```python
from build123d import *

# Parameters (mm, degrees)
F0_W     = 117
F0_H     = 15
F0_R     = 0.5
F1_DEPTH = 20
F2_W     = 10
F2_H     = 10
F3_DEPTH = 37


with BuildPart() as f1:
    # F0 (on Front) → F1 (new body)
    with BuildSketch(Plane.XZ):
        with Locations((67, 12)):
            Rectangle(F0_W, F0_H)
        with Locations((16, 12)):
            Circle(F0_R, mode=Mode.SUBTRACT)
        with Locations((40, 12)):
            Circle(F0_R, mode=Mode.SUBTRACT)
        with Locations((76, 12)):
            Circle(F0_R, mode=Mode.SUBTRACT)
        with Locations((106, 12)):
            Circle(F0_R, mode=Mode.SUBTRACT)
        with Locations((118, 12)):
            Circle(F0_R, mode=Mode.SUBTRACT)
    extrude(amount=F1_DEPTH)

    # F2 (on face) → F3 (cut)
    with BuildSketch(Plane.XY.offset(19.5)):
        with Locations((40, -10)):
            Rectangle(F2_W, F2_H)
        with Locations((106, -10)):
            Rectangle(F2_W, F2_H)
    extrude(amount=-F3_DEPTH, mode=Mode.SUBTRACT)


solid = f1.part
```
Here's how the part is built. I have some questions about the finished solid (model axes, mm). A direction names the side the tool comes from. Coordinates: 2 decimals unless noted, no trailing zeros. Order: outer loops, then holes, each group sorted by start corner. A loop starts at its lowest first (then second) coordinate and runs counter-clockwise, first axis right, second up.
1) Imagine slicing it at A-A on y = -9.25. List the corners of the cut face in (x, z) for me.
2) We'd pull the mould along Y, two halves only. Please class faces 1 (the face through (8.5, -10, 12)), 2 (the face through (41, -15, 12)), 3 (the face through (41, -5, 12)), 4 (the face through (66, 0, 12)): +Y half, -Y half, draft (parallel to the pull), parting line (faces both ways), or undercut.
3) Will this pin go through, and if not, where does the flat tip stop? pin 1 (8 mm diameter, centred on x = 41.5, z = 11.5, fed in from +Y).
4) I need wall thicknesses on line 1 (Z direction, x = 40, y = -4); line 2 (X direction, y = -5.25, z = 15); line 3 (Y direction, x = 109.5, z = 10.5). Which ranges of each line are inside material? Lowest first, please.
5) Which directions (+Z, -Z, +X, -X, +Y, -Y) give clear straight access to the entire face, cutting with the end or side of a thin tool? Please do faces 5 (the face through (66, -20, 12)), 6 (the face through (35, -10, 12)).
6) Imagine slicing it at B-B on z = 6.5. List the corners of the cut face in (x, y) for me, and give its area (3 significant figures).
Response values:
1. outline: (8.5, 4.5) - (35, 4.5) - (35, 19.5) - (8.5, 19.5) - close; (45, 4.5) - (101, 4.5) - (101, 19.5) - (45, 19.5) - close; (111, 4.5) - (125.5, 4.5) - (125.5, 19.5) - (111, 19.5) - close; hole circle Ø1 at (16, 12); hole circle Ø1 at (76, 12); hole circle Ø1 at (118, 12)
2. face 1: draft
2. face 2: undercut
2. face 3: undercut
2. face 4: +Y half
3. pin 1: stops at y = 0
4. line 1: z = 4.5 to 11.5, 12.5 to 19.5
4. line 2: x = 8.5 to 35, 45 to 101, 111 to 125.5
4. line 3: y = -20 to -15, -5 to 0
5. face 5: +Z, -Z, +X, -X, -Y
5. face 6: +Z, -Z
6. outline: (8.5, -20) - (125.5, -20) - (125.5, 0) - (8.5, 0) - close; hole (35, -15) - (45, -15) - (45, -5) - (35, -5) - close; hole (101, -15) - (111, -15) - (111, -5) - (101, -5) - close
6. area: 2,140 mm2
